Read the model definition and answer for the solid it produces. Units are mm, in the model's axes. A direction names the side the tool comes from. Coordinates: 2 decimals unless noted, no trailing zeros. Write each loop counter-clockwise with the first axis right and the second up, starting at its lowest first coordinate (ties: lowest second). Pieces come first, ordered by that corner, then holes.
Item 1: Each of these flat-tipped pins is pushed along its axis until it touches: P1, Ø8, axis at x = 58.5, z = 87, coming from the +Y side; P2, Ø2, axis at x = 22, y = 12.5, coming from the +Z side; P3, Ø6, axis at y = 13, z = 85.5, coming from the -X side; P4, Ø8, axis at x = 48.5, y = 13, coming from the +Z side. Where does it stop, or does it pass through?
Item 2: Determine the mould class of faces 5 (the face through (55.01, 10.14, 44.86)), 6 (the face through (10, 40, 15)) for opening direction X: released by +X, released by -X, zero draft, split by the parting line, or undercut.
Item 3: A tool of negligible diameter and unlimited length cuts with its end or side. For faces 1 (the face through (23.71, 10, 84)), 2 (the face through (66.654, 10.14, 44.761)), 3 (the face through (35, 16, 10)), 4 (the face through (35, 25, 20)), from which of +Z, -Z, +X, -X, +Y, -Y can it reach the whole face along a straight path? Write none if from no direction.
Item 4: Section D-D (z = 38) is taken. Give the vertices of the cut face in (x, y), then the cut area to 3 significant figures.
Item 5: Section B-B (x = 47) is taken. Give the vertices of the cut face in (y, z).
Item 6: Section A-A (y = 37) is taken. Give the vertices of the cut face in (x, z), then the cut area to 3 significant figures.
Item 7: Straight lines are drawn through the part: probe 1 along Z at (x, y) = (35.5, 12.5); probe 2 along Z at (x, y) = (55.5, 14); probe 3 along X at (y, z) = (7, 36). For each, find the intervals that lie inside material, in ascending order.
Item 8: Section C-C (z = 8.5) is taken. Give the vertices of the cut face in (x, y), then the cut area to 3 significant figures.
from build123d import *

# Parameters (mm, degrees)
SKETCH2_W           = 70
SKETCH2_H           = 40
BOSS_EXTRUDE1_DEPTH = 50
SKETCH3_W           = 40
SKETCH3_H           = 10
CUT_EXTRUDE1_DEPTH  = 40
SKETCH4_W           = 30
SKETCH4_H           = 40
CUT_EXTRUDE2_DEPTH  = 15
SKETCH5_W           = 70
SKETCH5_H           = 20
CUT_EXTRUDE3_DEPTH  = 20
BOSS_EXTRUDE2_DEPTH = 20
CUT_EXTRUDE4_DEPTH  = 124.693168769


with BuildPart() as part:
    # Sketch2 → Boss-Extrude1 (new body)
    with BuildSketch(Plane.XY):
        with Locations((35, 20)):
            Rectangle(SKETCH2_W, SKETCH2_H)
    extrude(amount=BOSS_EXTRUDE1_DEPTH)

    # Sketch3 → Cut-Extrude1 (cut)
    with BuildSketch(Plane(origin=(0, 40, 0), x_dir=(1, 0, 0), z_dir=(0, 1, 0))):
        with Locations((35, -5)):
            Rectangle(SKETCH3_W, SKETCH3_H)
    extrude(amount=-CUT_EXTRUDE1_DEPTH, mode=Mode.SUBTRACT)

    # Sketch4 → Cut-Extrude2 (cut)
    with BuildSketch(Plane(origin=(0, 40, 0), x_dir=(1, 0, 0), z_dir=(0, 1, 0))):
        with Locations((35, -30)):
            Rectangle(SKETCH4_W, SKETCH4_H)
    extrude(amount=-CUT_EXTRUDE2_DEPTH, mode=Mode.SUBTRACT)

    # Sketch5 → Cut-Extrude3 (cut)
    with BuildSketch(Plane(origin=(0, 40, 0), x_dir=(1, 0, 0), z_dir=(0, 1, 0))):
        with Locations((35, -40)):
            Rectangle(SKETCH5_W, SKETCH5_H)
    extrude(amount=-CUT_EXTRUDE3_DEPTH, mode=Mode.SUBTRACT)

    # Sketch6 → Boss-Extrude2 (add)
    with BuildSketch(Plane.XZ):
        Polygon((0, 50), (16.209807748, 99.268768354), (23.709807748, 99.268768354), (23.709807748, 69.268768354), (48.709807748, 69.268768354), (48.709807748, 100), (56.209807748, 100), (70, 50), align=None)
    extrude(amount=-BOSS_EXTRUDE2_DEPTH)

    # Sketch7 → Cut-Extrude4 (cut, through all)
    with BuildSketch(Plane(origin=(0, 20, 0), x_dir=(1, 0, 0), z_dir=(0, 1, 0))):
        with BuildLine():
            Line((5.284369051, -34.535416774), (12.378641305, -34.535416774))
            ThreePointArc((12.378641305, -34.535416774), (14.654162594, -36.810938063), (12.378641305, -39.086459352))
            Line((12.378641305, -39.086459352), (5.284369051, -39.086459352))
            ThreePointArc((5.284369051, -39.086459352), (3.008847762, -36.810938063), (5.284369051, -34.535416774))
        make_face()
        with BuildLine():
            Line((18.284369051, -34.535416774), (25.378641305, -34.535416774))
            ThreePointArc((25.378641305, -34.535416774), (27.654162594, -36.810938063), (25.378641305, -39.086459352))
            Line((25.378641305, -39.086459352), (18.284369051, -39.086459352))
            ThreePointArc((18.284369051, -39.086459352), (16.008847762, -36.810938063), (18.284369051, -34.535416774))
        make_face()
        with BuildLine():
            Line((31.284369051, -34.535416774), (38.378641305, -34.535416774))
            ThreePointArc((38.378641305, -34.535416774), (40.654162594, -36.810938063), (38.378641305, -39.086459352))
            Line((38.378641305, -39.086459352), (31.284369051, -39.086459352))
            ThreePointArc((31.284369051, -39.086459352), (29.008847762, -36.810938063), (31.284369051, -34.535416774))
        make_face()
        with BuildLine():
            Line((44.284369051, -34.535416774), (51.378641305, -34.535416774))
            ThreePointArc((51.378641305, -34.535416774), (53.654162594, -36.810938063), (51.378641305, -39.086459352))
            Line((51.378641305, -39.086459352), (44.284369051, -39.086459352))
            ThreePointArc((44.284369051, -39.086459352), (42.008847762, -36.810938063), (44.284369051, -34.535416774))
        make_face()
        with BuildLine():
            Line((57.284369051, -34.535416774), (64.378641305, -34.535416774))
            ThreePointArc((64.378641305, -34.535416774), (66.654162594, -36.810938063), (64.378641305, -39.086459352))
            Line((64.378641305, -39.086459352), (57.284369051, -39.086459352))
            ThreePointArc((57.284369051, -39.086459352), (55.008847762, -36.810938063), (57.284369051, -34.535416774))
        make_face()
        with BuildLine():
            Line((18.284369051, -42.535416774), (25.378641305, -42.535416774))
            ThreePointArc((25.378641305, -42.535416774), (27.654162594, -44.810938063), (25.378641305, -47.086459352))
            Line((25.378641305, -47.086459352), (18.284369051, -47.086459352))
            ThreePointArc((18.284369051, -47.086459352), (16.008847762, -44.810938063), (18.284369051, -42.535416774))
        make_face()
        with BuildLine():
            Line((31.284369051, -42.535416774), (38.378641305, -42.535416774))
            ThreePointArc((38.378641305, -42.535416774), (40.654162594, -44.810938063), (38.378641305, -47.086459352))
            Line((38.378641305, -47.086459352), (31.284369051, -47.086459352))
            ThreePointArc((31.284369051, -47.086459352), (29.008847762, -44.810938063), (31.284369051, -42.535416774))
        make_face()
        with BuildLine():
            Line((44.284369051, -42.535416774), (51.378641305, -42.535416774))
            ThreePointArc((51.378641305, -42.535416774), (53.654162594, -44.810938063), (51.378641305, -47.086459352))
            Line((51.378641305, -47.086459352), (44.284369051, -47.086459352))
            ThreePointArc((44.284369051, -47.086459352), (42.008847762, -44.810938063), (44.284369051, -42.535416774))
        make_face()
        with BuildLine():
            Line((57.284369051, -42.535416774), (64.378641305, -42.535416774))
            ThreePointArc((64.378641305, -42.535416774), (66.654162594, -44.810938063), (64.378641305, -47.086459352))
            Line((64.378641305, -47.086459352), (57.284369051, -47.086459352))
            ThreePointArc((57.284369051, -47.086459352), (55.008847762, -44.810938063), (57.284369051, -42.535416774))
        make_face()
        with BuildLine():
            Line((18.284369051, -50.535416774), (25.378641305, -50.535416774))
            ThreePointArc((25.378641305, -50.535416774), (27.654162594, -52.810938063), (25.378641305, -55.086459352))
            Line((25.378641305, -55.086459352), (18.284369051, -55.086459352))
            ThreePointArc((18.284369051, -55.086459352), (16.008847762, -52.810938063), (18.284369051, -50.535416774))
        make_face()
        with BuildLine():
            Line((31.284369051, -50.535416774), (38.378641305, -50.535416774))
            ThreePointArc((38.378641305, -50.535416774), (40.654162594, -52.810938063), (38.378641305, -55.086459352))
            Line((38.378641305, -55.086459352), (31.284369051, -55.086459352))
            ThreePointArc((31.284369051, -55.086459352), (29.008847762, -52.810938063), (31.284369051, -50.535416774))
        make_face()
        with BuildLine():
            Line((44.284369051, -50.535416774), (51.378641305, -50.535416774))
            ThreePointArc((51.378641305, -50.535416774), (53.654162594, -52.810938063), (51.378641305, -55.086459352))
            Line((51.378641305, -55.086459352), (44.284369051, -55.086459352))
            ThreePointArc((44.284369051, -55.086459352), (42.008847762, -52.810938063), (44.284369051, -50.535416774))
        make_face()
        with BuildLine():
            Line((57.284369051, -50.535416774), (64.378641305, -50.535416774))
            ThreePointArc((64.378641305, -50.535416774), (66.654162594, -52.810938063), (64.378641305, -55.086459352))
            Line((64.378641305, -55.086459352), (57.284369051, -55.086459352))
            ThreePointArc((57.284369051, -55.086459352), (55.008847762, -52.810938063), (57.284369051, -50.535416774))
        make_face()
        with BuildLine():
            Line((5.284369051, -42.535416774), (12.378641305, -42.535416774))
            ThreePointArc((12.378641305, -42.535416774), (14.654162594, -44.810938063), (12.378641305, -47.086459352))
            Line((12.378641305, -47.086459352), (5.284369051, -47.086459352))
            ThreePointArc((5.284369051, -47.086459352), (3.008847762, -44.810938063), (5.284369051, -42.535416774))
        make_face()
        with BuildLine():
            Line((5.284369051, -50.535416774), (12.378641305, -50.535416774))
            ThreePointArc((12.378641305, -50.535416774), (14.654162594, -52.810938063), (12.378641305, -55.086459352))
            Line((12.378641305, -55.086459352), (5.284369051, -55.086459352))
            ThreePointArc((5.284369051, -55.086459352), (3.008847762, -52.810938063), (5.284369051, -50.535416774))
        make_face()
    extrude(amount=-CUT_EXTRUDE4_DEPTH, mode=Mode.SUBTRACT)


solid = part.part
Established:
1. P1: stops at y = 20
1. P2: stops at z = 99.27
1. P3: stops at x = 10.69
1. P4: stops at z = 100
2. face 5: undercut
2. face 6: zero draft
3. face 1: +Z, +Y, -Y
3. face 2: +Y, -Y
3. face 3: -Z, +Y, -Y
3. face 4: +Z, -Z, +Y
4. outline: (0, 0) - (3.34, 0) - (3.34, 20) - (0, 20) - close; (14.32, 0) - (16.34, 0) - (16.34, 20) - (14.32, 20) - close; (27.32, 0) - (29.34, 0) - (29.34, 20) - (27.32, 20) - close; (40.32, 0) - (42.34, 0) - (42.34, 20) - (40.32, 20) - close; (53.32, 0) - (55.34, 0) - (55.34, 20) - (53.32, 20) - close; (66.32, 0) - (70, 0) - (70, 20) - (66.32, 20) - close
4. area: 303 mm2
5. outline: (0, 10) - (25, 10) - (25, 30) - (20, 30) - (20, 34.54) - (0, 34.54) - close; (0, 39.09) - (20, 39.09) - (20, 42.54) - (0, 42.54) - close; (0, 47.09) - (20, 47.09) - (20, 50.54) - (0, 50.54) - close; (0, 55.09) - (20, 55.09) - (20, 69.27) - (0, 69.27) - close
6. outline: (0, 0) - (15, 0) - (15, 10) - (20, 10) - (20, 30) - (0, 30) - close; (50, 10) - (55, 10) - (55, 0) - (70, 0) - (70, 30) - (50, 30) - close
6. area: 1,100 mm2
7. probe 1: z = 10 to 34.54, 39.09 to 42.54, 47.09 to 50.54, 55.09 to 69.27
7. probe 2: z = 0 to 35.4, 38.22 to 43.4, 46.22 to 51.4, 54.22 to 100
7. probe 3: x = 0 to 3.16, 14.5 to 16.16, 27.5 to 29.16, 40.5 to 42.16, 53.5 to 55.16, 66.5 to 70
8. outline: (0, 0) - (15, 0) - (15, 40) - (0, 40) - close; (55, 0) - (70, 0) - (70, 40) - (55, 40) - close
8. area: 1,200 mm2
